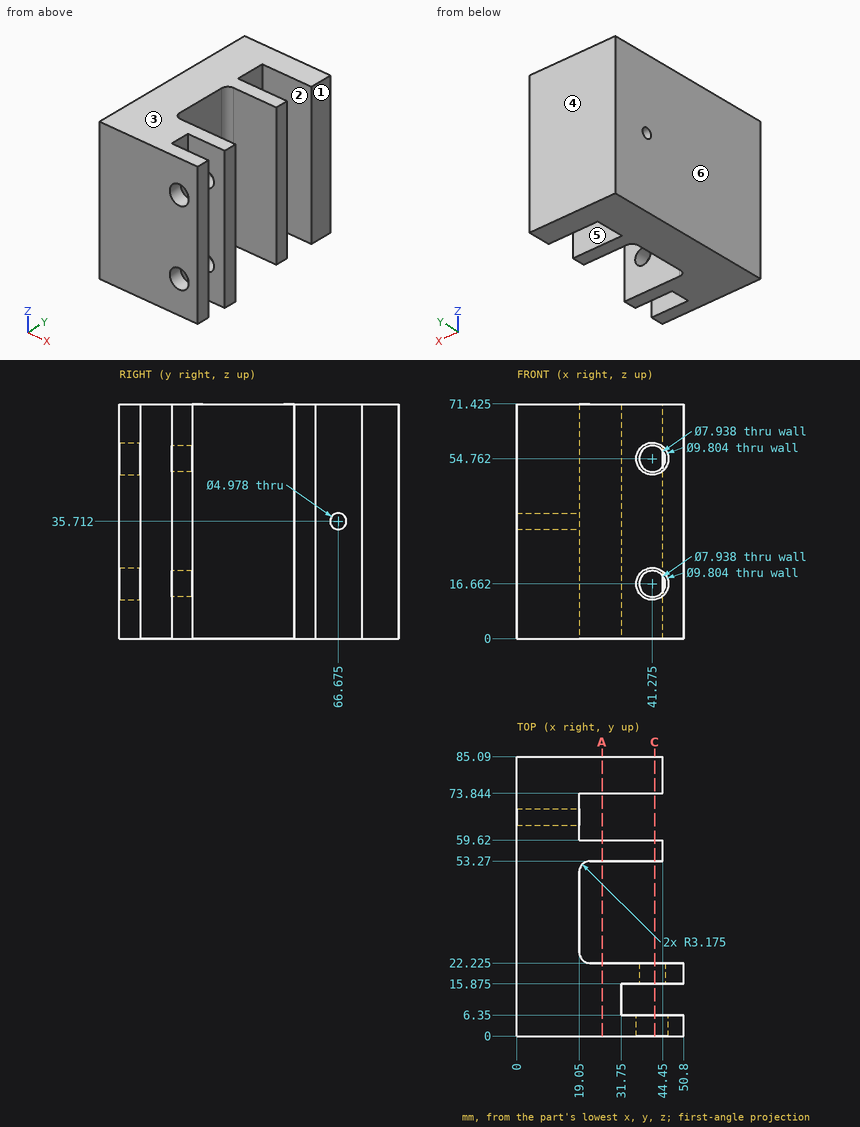
Part print with two shaded views. Sizes in mm from the minimum x, y, z corner. A direction names the side the tool comes from. Give positions to 0.01 mm unless a question says otherwise; leave off trailing zeros. Write each loop counter-clockwise with the first axis right and the second up, starting at its lowest first coordinate (ties: lowest second). Pieces come first, ordered by that corner, then holes.
1) Pin check, flat tips, straight feed: pin 1 (9 mm diameter, centred on x = 41.28, z = 54.76, fed in from -Y) (1 decimal); pin 2 (3.5 mm diameter, centred on y = 80.5, z = 43.5, fed in from +X); pin 3 (5 mm diameter, centred on x = 22, y = 65, fed in from +Z); pin 4 (1.5 mm diameter, centred on x = 40.5, z = 56, fed in from -Y). Stop position of each tip, or through.
Resolved:
pin 1: stops at y = 15.9
pin 2: stops at x = 44.45
pin 3: passes through
pin 4: stops at y = 53.27
2) Cut at A-A on x = 26. Write the cut outline in (y, z) (1 decimal).
Resolved:
outline: (0, 0) - (22.2, 0) - (22.2, 71.4) - (0, 71.4) - close; (53.3, 0) - (59.6, 0) - (59.6, 71.4) - (53.3, 71.4) - close; (73.8, 0) - (85.1, 0) - (85.1, 71.4) - (73.8, 71.4) - close
3) Two-plate mould, pull along Y, no slides. Class the marked faces 4, 5 and 6: released by +Y, released by -Y, zero draft, split by the parting line, or undercut.
Resolved:
face 4: released by +Y
face 5: undercut
face 6: zero draft
4) Which spindle directions (+Z, -Z, +X, -X, +Y, -Y) get a long thin tool onto all of the face, cutting with end or side? Do the marked faces 1, 2 and 3. Say none if no direction does.
Resolved:
face 1: +Z, -Z, +X, +Y
face 2: +Z, -Z, +X
face 3: +Z, +X, -X, +Y, -Y
5) Cut at C-C on x = 42. State how many separate pieces and enclosed holes the cut face has, then the cut area to 3 significant figures.
Resolved:
separate pieces: 8
enclosed holes: 0
area: 1,940 mm2
6) Probe L1, parallel to Y at x = 24, z = 4.5 (1 decimal); L2, parallel to Y at x = 9, z = 36; L3, parallel to X at y = 33.5, z = 48.5. List the from-to ranges inside material, lowest first.
Resolved:
L1: y = 0 to 22.2, 53.3 to 59.6, 73.8 to 85.1
L2: y = 0 to 64.2, 69.15 to 85.09
L3: x = 0 to 19.05
